Part model, mm, in its own coordinate system. A direction names the side the tool comes from. Round coordinates to 2 decimals unless told otherwise and drop trailing zeros. Loops run counter-clockwise (first coordinate to the right, second up) from the corner with the lowest first, then second, coordinate; pieces in that order, holes last.
1) Probe line 1 (X direction, y = 0, z = -7.5); line 2 (Y direction, x = 0.75, z = -4); line 3 (X direction, y = 0.5, z = -8.25). List the from-to ranges inside material, lowest first.
2) Band-saw the part on A-A, the plane x = 0. Write the cut outline in (y, z), then the cut area to 3 significant figures.
3) Mould opens along X. For faces 1 (the flat face through (-1.3, -1.3, -12)), 2 (the cylindrical face through (0.07, -1.5, -6.08)), 3 (the cylindrical face through (-2.44, -0.54, -0.54)) say: +X half, -X half, draft (parallel to the pull), parting line (faces both ways), or undercut.
4) Band-saw the part on D-D, the plane x = 2. Write the cut outline in (y, z), then the cut area to 3 significant figures.
5) 3-axis set-ups, long thin cutter, end or side, ignore diameter. For faces 4 (the cylindrical face through (0, -3, -11)), 5 (the flat face through (0, 2, 0)), 6 (the cylindrical face through (-2.44, -0.54, -7.97)): which of +Z, -Z, +X, -X, +Y, -Y reach the whole face in a straight line?
6) Band-saw the part on C-C, the plane z = -8.75. Write the cut outline in (x, y), then the cut area to 3 significant figures.
7) Drop flat-ended pins along their axis: P1, Ø1, axis at x = 0.5, z = -4.5, coming from the +Y side; P2, Ø1, axis at y = 0.5, z = -10, coming from the -X side. Give the stop position or say it passes through.
from build123d import *


with BuildPart() as part:
    # Sketch1 → Revolve1 (revolve)
    with BuildSketch(Plane(origin=(0, 0, 0), x_dir=(0, 0, -1), z_dir=(1, 0, 0))):
        with BuildLine():
            Line((0.388232597, 1.5), (6.712787917, 1.5))
            ThreePointArc((6.712787917, 1.5), (6.400595054, 2.031506006), (6, 2.5))
            ThreePointArc((6, 2.5), (3.550510257, 3.5), (1.101020514, 2.5))
            ThreePointArc((1.101020514, 2.5), (0.700425461, 2.031506006), (0.388232597, 1.5))
        make_face()
        with BuildLine():
            Line((6.712787917, 1.5), (12, 1.5))
            Line((12, 1.5), (12, 3))
            Line((12, 3), (10, 3))
            Line((10, 3), (10, 2.5))
            Line((10, 2.5), (6, 2.5))
            ThreePointArc((6, 2.5), (6.400595054, 2.031506006), (6.712787917, 1.5))
        make_face()
        with BuildLine():
            Line((0, 1.5), (0.388232597, 1.5))
            ThreePointArc((0.388232597, 1.5), (0.700425461, 2.031506006), (1.101020514, 2.5))
            Line((1.101020514, 2.5), (0, 2.5))
            Line((0, 2.5), (0, 1.5))
        make_face()
    revolve(axis=Axis((0, 0, 0), (0, 0, -1)))


solid = part.part
Reported:
1. line 1: x = -2.5 to -1.5, 1.5 to 2.5
1. line 2: y = -3.39 to -1.3, 1.3 to 3.39
1. line 3: x = -2.45 to -1.41, 1.41 to 2.45
2. outline: (-3, -12) - (-1.5, -12) - (-1.5, 0) - (-2.5, 0) - (-2.5, -1.1) arc R3.5 ccw to (-2.5, -6) - (-2.5, -10) - (-3, -10) - close; (1.5, -12) - (3, -12) - (3, -10) - (2.5, -10) - (2.5, -6) arc R3.5 ccw to (2.5, -1.1) - (2.5, 0) - (1.5, 0) - close
2. area: 32.7 mm2
3. face 1: draft
3. face 2: undercut
3. face 3: parting line
4. outline: (-2.24, -12) - (2.24, -12) - (2.24, -10) - (1.5, -10) - (1.5, -6) arc R2.87 ccw to (1.5, -1.1) - (1.5, 0) - (-1.5, 0) - (-1.5, -1.1) arc R2.87 ccw to (-1.5, -6) - (-1.5, -10) - (-2.24, -10) - close
4. area: 48.4 mm2
5. face 4: -Z
5. face 5: +Z, +X, -X, +Y, -Y
5. face 6: none
6. outline: circle Ø5 at (0, 0); hole circle Ø3 at (0, 0)
6. area: 12.6 mm2
7. P1: stops at y = 3.45
7. P2: stops at x = -3
